Design review of the part built by this model. Coordinates are the model's own, in mm. Face numbers are marked on the shaded views. A direction names the side the tool comes from. Give positions to 0.01 mm unless a question says otherwise; leave off trailing zeros. Write each loop counter-clockwise with the first axis right and the second up, starting at its lowest first coordinate (ties: lowest second). Pieces come first, ordered by that corner, then holes. Notation, with made-up numbers: (14.25, 5.25) - (51.25, 5.25) arc R9 cw to (51.25, 9.25) - close; hole circle Ø8 at (-8.75, 75.25). An arc over 180 degrees is marked (long way). Use a Markdown table: item, result. Add a question column.
```python
from build123d import *

# Parameters (mm, degrees)
F0_W      = 226.3691648841
F0_H      = 109.7707115114
F1_DEPTH  = 62
F2_W      = 219.8443636298
F2_H      = 100.2121046185
F3_DEPTH  = 13
F4_W      = 6.5248012543
F4_H      = 60.6752280146
F5_DEPTH  = 22
F7_DEPTH  = 20
F8_R      = 5
F9_R      = 5
F10_R     = 5
F11_R     = 5
F12_W     = 79.6035556123
F12_H     = 8.4695416391
F13_DEPTH = 25


with BuildPart() as f1:
    # F0 (on Top) → F1 (new body)
    with BuildSketch(Plane.XY):
        with Locations((-2.5108121336, -0.4434902221)):
            Rectangle(F0_W, F0_H)
    extrude(amount=F1_DEPTH)

    # F2 (on face) → F3 (cut)
    with BuildSketch(Plane.XY.offset(62)):
        with Locations((0.7515884936, -5.2227936685)):
            Rectangle(F2_W, F2_H)
    extrude(amount=-F3_DEPTH, mode=Mode.SUBTRACT)

    # F4 (on face) → F5 (cut)
    with BuildSketch(Plane.XY.offset(62)):
        with Locations((-112.4329939485, 8.6751645431)):
            Rectangle(F4_W, F4_H)
    extrude(amount=-F5_DEPTH, mode=Mode.SUBTRACT)

    # F6 (on face) → F7 (cut)
    with BuildSketch(Plane.XY.offset(49)):
        Polygon((95.4916924238, 44.8832586408), (-109.1705933213, 44.8832586408), (-109.1705933213, 39.0127785504), (-109.1705933213, -21.6624494642), (-109.1705933213, -44.0085157752), (95.4916924238, -44.0085157752), align=None)
    extrude(amount=-F7_DEPTH, mode=Mode.SUBTRACT)

    # F8
    f8_edges = [f1.edges().sort_by_distance(p)[0] for p in [
        (95.491692, 44.883259, 39),
    ]]
    fillet(f8_edges, radius=F8_R)

    # F9
    f9_edges = [f1.edges().sort_by_distance(p)[0] for p in [
        (95.491692, -44.008516, 39),
    ]]
    fillet(f9_edges, radius=F9_R)

    # F10
    f10_edges = [f1.edges().sort_by_distance(p)[0] for p in [
        (-109.170593, -44.008516, 39),
    ]]
    fillet(f10_edges, radius=F10_R)

    # F11
    f11_edges = [f1.edges().sort_by_distance(p)[0] for p in [
        (-109.170593, 44.883259, 45.5),
    ]]
    fillet(f11_edges, radius=F11_R)

    # F12 (on face) → F13 (cut)
    with BuildSketch(Plane(origin=(0, 54.4418655336, 0), x_dir=(-1, 0, 0), z_dir=(0, 1, 0))):
        with Locations((54.2112276889, 57.7652291805)):
            Rectangle(F12_W, F12_H)
    extrude(amount=-F13_DEPTH, mode=Mode.SUBTRACT)


solid = f1.part
```
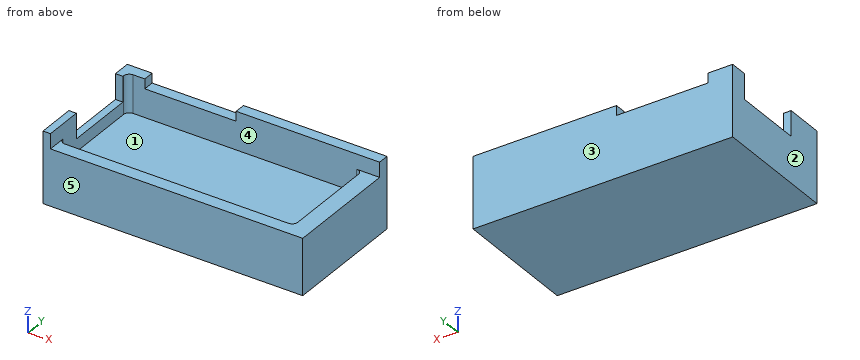
(1) Mouldability with a two-part tool opening along Y and no side actions: class the marked faces 1, 2 and 3 as +Y half, -Y half, draft (parallel to the pull), parting line (faces both ways), or undercut.
(2) Add section D-D (x = -17.5). State the section outline as (y, z) points, and give its area (3 significant figures).
(3) Add section C-C (z = 45.5). State the section outline as (x, y) points.
(4) Add section B-B (y = 2). State the section outline as (x, z) points, and give its area (3 significant figures).
(5) Tool access review of the marked faces 4 and 5: name each direction out of +Z, -Z, +X, -X, +Y, -Y from which nothing blocks a thin tool from reaching the whole face with its end or side.
(6) Insertion check: pin 1 (1 mm diameter, centred on x = 27, y = -34.5, fed in from +Z); pin 2 (7 mm diameter, centred on x = -112, y = 16, fed in from +Z); pin 3 (3 mm diameter, centred on x = -48, y = 49, fed in from +Z). Each pin has a flat end and moves straight along its axis. Give the tip position at first contact, or say it passes through.
(7) Add section A-A (z = 57.5). State the section outline as (x, y) points.
(8) For line 1 along Y through (x, z) = (91, 43); line 2 along X through (y, z) = (-36.5, 33.5); line 3 along X through (y, z) = (-43, 49.5), list the stretches that pass through material, from the lowest coordinate up.
Answers follow:
| question | item | result |
|---|---|---|
| 1 | face 1 | undercut |
| 1 | face 2 | draft |
| 1 | face 3 | +Y half |
| 2 | outline | (-55.33, 0) - (54.44, 0) - (54.44, 53.53) - (44.88, 53.53) - (44.88, 29) - (-44.01, 29) - (-44.01, 49) - (-55.33, 49) - close |
| 2 | area | 3,640 mm^2 |
| 3 | outline | (-115.7, -55.33) - (110.67, -55.33) - (110.67, 54.44) - (-115.7, 54.44) - (-115.7, 39.01) - (-109.17, 39.01) - (-109.17, 39.88) arc R5 cw to (-104.17, 44.88) - (90.49, 44.88) arc R5 cw to (95.49, 39.88) - (95.49, -39.01) arc R5 cw to (90.49, -44.01) - (-104.17, -44.01) arc R5 cw to (-109.17, -39.01) - (-109.17, -21.66) - (-115.7, -21.66) - close |
| 4 | outline | (-115.7, 0) - (110.67, 0) - (110.67, 49) - (95.49, 49) - (95.49, 29) - (-109.17, 29) - (-109.17, 40) - (-115.7, 40) - close |
| 4 | area | 6,940 mm^2 |
| 5 | face 4 | +Z |
| 5 | face 5 | +Z, -Z, +X, -X, -Y |
| 6 | pin 1 | z = 29 |
| 6 | pin 2 | z = 40 |
| 6 | pin 3 | z = 53.53 |
| 7 | outline | (-115.7, -55.33) - (-109.17, -55.33) - (-109.17, -21.66) - (-115.7, -21.66) - close; (-115.7, 39.01) - (-109.17, 39.01) - (-109.17, 39.88) arc R5 cw to (-104.17, 44.88) - (-94.01, 44.88) - (-94.01, 54.44) - (-115.7, 54.44) - close; (-14.41, 44.88) - (110.67, 44.88) - (110.67, 54.44) - (-14.41, 54.44) - close |
| 8 | line 1 | -55.33 to -43.98, 44.86 to 54.44 |
| 8 | line 2 | -115.7 to -109.17, 95.49 to 110.67 |
| 8 | line 3 | -115.7 to -109.17 |
